Part model, mm, in its own coordinate system. A direction names the side the tool comes from. Coordinates: 2 decimals unless noted, no trailing zeros. Loops run counter-clockwise (first coordinate to the right, second up) from the corner with the lowest first, then second, coordinate; pieces in that order, holes last. Notation, with made-up numbers: M 79.25,-38.5 L 88.25,-38.5 A26 ccw 88.25,-11.5 Z; hole C 37.5,13 d5. An arc over 180 degrees is marked long. Answer as a JSON object with one key per item and string values. Group by question number.
1. Drop flat-ended pins along their axis: pin 1 Ø4 at (x, y) = (-28, 0) entering from -Z; pin 2 Ø1.5 at (y, z) = (-8, 49) entering from +X; pin 3 Ø4 at (x, z) = (30.5, 46.5) entering from -Y. Give the stop position or say it passes through.
2. Mould opens along Z. For faces 4 (the face through (-2.87, 34.52, 2.64)), 5 (the face through (6.35, 0, -29)), 6 (the face through (12, 6.35, 1)) say: released by +Z, released by -Z, zero draft, split by the parting line, or undercut.
3. 3-axis set-ups, long thin cutter, end or side, ignore diameter. For faces 1 (the face through (-6.35, 0, -28)), 2 (the face through (0, 63.5, 0)), 3 (the face through (-2.87, -35.33, 2.64)): which of +Z, -Z, +X, -X, +Y, -Y reach the whole face in a straight line?
4. Drill centre lines: L1, parallel to X at y = -2, z = 12.5; L2, parallel to Z at x = 34, y = 3; L3, parallel to Z at x = 43, y = 2.5. Where is each one in solid material? Low to high.
5. Saw through at C-C on y = -36. Write the cut outline in (x, z), then the cut area to 3 significant figures.
6. Saw through at D-D on x = -25. Count the separate pieces of the cut face and the enclosed holes in it, then the cut area to 3 significant figures.
from build123d import *

# Parameters (mm, degrees)
F0_R     = 63.5
F0_R_2   = 3.81
F1_DEPTH = 6.35
F2_R     = 6.34999
F3_R     = 3.9002189419
F4_DEPTH = 63.5


# Not quite as in the source:
# - a fillet or chamfer is up to 0.001 mm smaller than in the source, because OpenCascade refuses the exact size


with BuildPart() as f1:
    # F0 (on Front) → F1 (new body, symmetric)
    with BuildSketch(Plane.XZ):
        Circle(F0_R)
        with BuildLine():
            ThreePointArc((-6.35, -50.4015624758), (-35.9210244843, -35.9210244843), (-50.4015624758, -6.35))
            Line((-50.4015624758, -6.35), (-6.35, -6.35))
            Line((-6.35, -6.35), (-6.35, -50.4015624758))
        make_face(mode=Mode.SUBTRACT)
        with BuildLine():
            Line((6.35, -50.4015624758), (6.35, -6.35))
            Line((6.35, -6.35), (50.4015624758, -6.35))
            ThreePointArc((50.4015624758, -6.35), (35.9210244843, -35.9210244843), (6.35, -50.4015624758))
        make_face(mode=Mode.SUBTRACT)
        with BuildLine():
            Line((-6.3499999233, 50.4015624854), (-6.3499999233, 6.35))
            Line((-6.3499999233, 6.35), (-50.4015624758, 6.35))
            ThreePointArc((-50.4015624758, 6.35), (-35.9210244569, 35.9210245116), (-6.3499999233, 50.4015624854))
        make_face(mode=Mode.SUBTRACT)
        Circle(F0_R_2, mode=Mode.SUBTRACT)
        with BuildLine():
            Line((50.4015624854, 6.3499999233), (6.35, 6.3499999233))
            Line((6.35, 6.3499999233), (6.35, 50.4015624758))
            ThreePointArc((6.35, 50.4015624758), (35.9210245116, 35.9210244569), (50.4015624854, 6.3499999233))
        make_face(mode=Mode.SUBTRACT)
    extrude(amount=F1_DEPTH, both=True)

    # F2 (radius 6.35 in the source; OpenCascade refuses exactly that, so slightly less here)
    f2_edges = [f1.edges().sort_by_distance(p)[0] for p in [
        (-63.5, 6.35, 0),
        (63.5, 0, 0),
        (-63.5, -6.35, 0),
    ]]
    fillet(f2_edges, radius=F2_R)

    # F3 (on Front) → F4 (join, symmetric)
    with BuildSketch(Plane.XZ):
        with Locations((4.138e-07, 0)):
            Circle(F3_R)
    extrude(amount=F4_DEPTH, both=True)


solid = f1.part
Outcome:
{
 "1": {"pin 1": "stops at z = -57.93", "pin 2": "passes through", "pin 3": "stops at y = -6.35"},
 "2": {"face 4": "split by the parting line", "face 5": "undercut", "face 6": "zero draft"},
 "3": {"face 1": "+Y, -Y", "face 2": "+Z, -Z, +X, -X, +Y", "face 3": "-Y"},
 "4": {"L1": "x = -61.93 to -49.24, -6.35 to 6.35, 49.24 to 61.93", "L2": "z = -52.74 to -37.74, -6.35 to 6.35, 37.74 to 52.74", "L3": "z = -46.03 to -27.05, -6.35 to 6.35, 27.05 to 46.03"},
 "5": {"outline": "C 0,0 d7.8", "area": "47.8 mm²"},
 "6": {"separate pieces": "3", "enclosed holes": "0", "area": "483 mm²"}
}
